Could you check a few things on this drawing? It's one solid part, dimensions in mm from its lowest x, y, z. Give positions to 0.01 mm unless a question says otherwise; leave off trailing zeros. Order: outer loops, then holes, each group sorted by start corner. A loop starts at its lowest first (then second) coordinate and runs counter-clockwise, first axis right, second up. Notation, with made-up numbers: (72, -5.75) -> (77, -5.75) arc R25 cw to (77, 15.25) -> close; hole circle Ø4 at (-1.5, 72). An arc over 180 degrees is marked (long way). Answer as CSV lines item,"result".
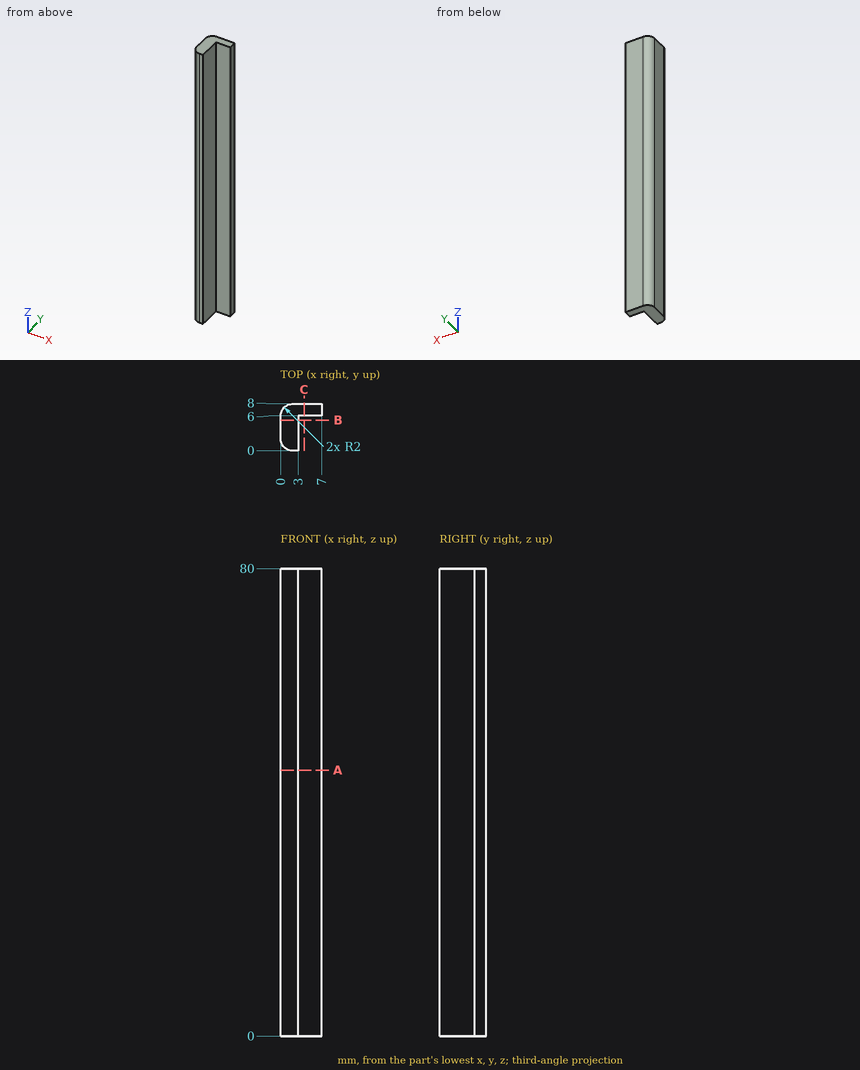
Item 1: Imagine slicing it at C-C, the plane x = 4. Please give me the cut outline in (y, z), then the cut area to 3 significant figures.
Numbers:
outline,"(6, 0) -> (8, 0) -> (8, 80) -> (6, 80) -> close"
area,"160 mm²"
Item 2: Please list where these lines run through material, in increasing order: line 1 along X through (y, z) = (5, 38); line 2 along Y through (x, z) = (4, 35.5); line 3 along X through (y, z) = (6.25, 64).
Numbers:
line 1,"x = 0 to 3"
line 2,"y = 6 to 8"
line 3,"x = 0.02 to 7"
Item 3: For pin 1 (1.5 mm diameter, centred on y = 2.5, z = 8.5, fed in from +X), with a flat end and sliding along its axis, tell me the tip position at first contact or that it passes through.
Numbers:
pin 1,"stops at x = 3"
Item 4: Imagine slicing it at A-A, the plane z = 45.5. Please give me the cut outline in (x, y).
Numbers:
outline,"(0, 2) arc R2 ccw to (2, 0) -> (3, 0) -> (3, 6) -> (7, 6) -> (7, 8) -> (2, 8) arc R2 ccw to (0, 6) -> close"
Item 5: Imagine slicing it at B-B, the plane y = 5.25. Please give me the cut outline in (x, z).
Numbers:
outline,"(0, 0) -> (3, 0) -> (3, 80) -> (0, 80) -> close"
